from build123d import *

# Parameters (mm, degrees)
PIPESKETCH_R   = 6.35
PIPESKETCH_R_2 = 5.1054


with BuildPart() as part:
    # ThinSweep: sweep along a curve in space
    with BuildLine() as thinsweep_path:
        Line((0, 0, 0), (0, 0, 45.224833485))
        ThreePointArc((0, 0, 45.224833485), (6.49695017, -9.072931676, 72.165601848), (22.181975386, -30.97692638, 83.324833485))
        Line((22.181975386, -30.97692638, 83.324833485), (259.82889592, -362.848684139, 83.324833485))
        ThreePointArc((282.010871306, -393.825610519, 45.224833485), (275.513921135, -384.752678843, 72.165601848), (259.82889592, -362.848684139, 83.324833485))
        Line((282.010871306, -393.825610519, -400.347253913), (282.010871306, -393.825610519, 45.224833485))
    # PipeSketch → ThinSweep (sweep)
    with BuildSketch(Plane.XY):
        Circle(PIPESKETCH_R)
        Circle(PIPESKETCH_R_2, mode=Mode.SUBTRACT)
    sweep(path=thinsweep_path.line)


solid = part.part
Model file for the job. Use its own axes, mm. Coordinates: 2 decimals unless noted, no trailing zeros. Loops run counter-clockwise (first coordinate to the right, second up) from the corner with the lowest first, then second, coordinate; pieces in that order, holes last. Notation, with made-up numbers: (53.5, -32) -> (91.5, -32) arc R15 ccw to (91.5, -6) -> close; hole circle Ø9 at (78.25, 74). An arc over 180 degrees is marked (long way). Use one line per item in the form item = value. Start each with the question number.
(1) Flat gauge pin, fed straight in: pin 1 (10 mm diameter, centred on x = 0, y = -0.5, fed in from -Z). Where does the tip first touch, or does it go through?
(2) Pull direction Z, two halves, no side cores. Call faces 1 (the cylindrical face through (144.861, -197.666, 78.989)), 2 (the cylindrical face through (280.23, -399.92, -180.68)), 3 (the cylindrical face through (145.103, -197.493, 88.925)): pulls with the +Z half, pulls with the -Z half, needs draft (parallel to the pull), parting line crosses it, or undercut.
(3) Probe probe 1 along Y at (x, z) = (0, 15.5). List the from-to ranges inside material, lowest first. Write a range as from..to.
(4) Cut at A-A on z = 28.5. Give the cut face in (x, y), and give its area (3 significant figures).
(5) Cut at B-B on z = -357. Give the cut face in (x, y).
Values:
q1.pin_1 = 0
q2.face_1 = undercut
q2.face_2 = needs draft
q2.face_3 = parting line crosses it
q3.probe_1 = -6.35..-5.11, 5.11..6.35
q4.outline = circle Ø12.7 at (0, 0); circle Ø12.7 at (282.01, -393.83); hole circle Ø10.21 at (0, 0); hole circle Ø10.21 at (282.01, -393.83)
q4.area = 89.6 mm2
q5.outline = circle Ø12.7 at (282.01, -393.83); hole circle Ø10.21 at (282.01, -393.83)
